The listing builds one solid part. Answer for the finished solid, in the listing's coordinates (mm). A direction names the side the tool comes from. Give positions to 0.01 mm unless a question says otherwise; leave off trailing zeros. Write each loop counter-clockwise with the first axis right and the second up, starting at its lowest first coordinate (ties: lowest second). Pieces come first, ordered by that corner, then holes. Notation, with made-up numbers: (64, 28) - (116, 28) arc R20 ccw to (116, 66) - close; hole circle Ø5 at (0, 53.5). An arc over 180 degrees is marked (long way). Answer in a Markdown table with one row per item. Add a question column.
Autodesk Inventor part; units mm, degrees
ref_plane "YZ Plane" through (0, 0, 0) normal (1, 0, 0) x (0, 1, 0)
ref_plane "XZ Plane" through (0, 0, 0) normal (0, 1, 0) x (-1, 0, 0)
ref_plane "XY Plane" through (0, 0, 0) normal (0, 0, 1) x (1, 0, 0)
sketch "Sketch1" plane through (0, 0, 0) normal (1, 0, 0) x (0, 1, 0)
  line L0 (0, 0) -> (3.95, 0)
  line L1 (3.95, 0) -> (3.95, 0.1833)
  line L2 (3.95, 0.1833) -> (3.7667, 0.3667)
  line L3 (3.7667, 0.3667) -> (3.7667, 0.55)
  line L4 (3.7667, 0.55) -> (6.555, 0.55)
  line L5 (6.555, 0.55) -> (6.555, 1.1)
  line L6 (6.555, 1.1) -> (3.115, 1.1)
  line L7 (3.115, 1.1) -> (3.115, 1.2)
  arc A0 (3.115, 1.3908) -> (3.115, 1.2) centre (3.145, 1.2954) ccw
  line L8 (3.115, 1.6816) -> (3.115, 5.1)
  line L9 (3.115, 5.1) -> (0, 5.1)
  line L10 (0, 5.1) -> (0, 0)
  arc A1 (3.115, 1.6816) -> (3.115, 1.4908) centre (3.145, 1.5862) ccw
  line L11 (3.115, 1.3908) -> (3.115, 1.4908)
  dimension "d0" = 7.9
  dimension "d1" = 1.1
  dimension "d2" = 6.23
  dimension "d3" = 13.11
  dimension "d4" = 4
  dimension "d5" = 0.1
  dimension "d6" = 0.55
  dimension "d7" = 0.1833
  dimension "d8" = 0.1833
  dimension "d9" = 0.1833
  dimension "d10" = 0.03
  dimension "d11" = 0.1
  dimension "d12" = 0.1
revolve "Revolution1" add sketch "Sketch1" angle 360 about axis through (0, 0, 5.1) along (0, 0, -1)
sketch "Sketch2" plane through (0, 0, 0.55) normal (0, 0, -1) x (-1, 0, 0)
  line L0 (1.1709, 4.37) -> (3.1991, 3.1991)
  line L1 (3.1991, 3.1991) -> (4.37, 1.1709)
  line L2 (4.37, 1.1709) -> (4.37, -1.1709)
  line L3 (4.37, -1.1709) -> (3.1991, -3.1991)
  line L4 (3.1991, -3.1991) -> (1.1709, -4.37)
  line L5 (1.1709, -4.37) -> (-1.1709, -4.37)
  line L6 (-1.1709, -4.37) -> (-3.1991, -3.1991)
  line L7 (-3.1991, -3.1991) -> (-4.37, -1.1709)
  line L8 (-4.37, -1.1709) -> (-4.37, 1.1709)
  line L9 (-4.37, 1.1709) -> (-3.1991, 3.1991)
  line L10 (-3.1991, 3.1991) -> (-1.1709, 4.37)
  line L11 (-1.1709, 4.37) -> (1.1709, 4.37)
  circle A0 centre (0, 0) radius 6.555
  dimension "d16" = 8.74
extrude "Extrusion1" cut sketch "Sketch2" against normal through all
hole "Hole1" at (0, 0, 5.1) direction (0, 0, -1) diameter 3.242 end through all countersink diameter 4.2 countersink angle 120
hole "Hole2" [suppressed]
equation "\"d0\" = C_"
equation "\"d1\" = A_"
equation "\"d2\" = B"
equation "\"d3\" = 1.5 * H_"
equation "\"d4\" = Length_Code"
equation "\"d5\" = Mark_1"
equation "\"d6\" = 0.5 * A_"
equation "\"d7\" = 0.166667 * A_"
equation "\"d8\" = 0.166667 * A_"
equation "\"d9\" = 0.166667 * A_"
equation "\"d10\" = Mark_2"
equation "\"d11\" = Mark_1"
equation "\"d12\" = Mark_1"
equation "\"d13\" = T_"
equation "\"d14\" = 1.05 * Thread"
equation "\"d53\" = Length_Code"
equation "\"d18\" = 1.05 * Thread"
equation "\"d20\" = T_"
equation "\"d16\" = H_"
equation "\"Length_Code\" = 4"
equation "\"T_\" = 4"
equation "\"A_\" = 1.1"
equation "\"B\" = 6.23"
equation "\"C_\" = 7.9"
equation "\"H_\" = 8.74"
equation "\"Mark_1\" = 0.1"
equation "\"Mark_2\" = 0.03"
equation "\"Thread\" = 4"
equation "\"Min_Thick\" = 1.6"
equation "\"B_Hole\" = 7.92"
equation "\"Min_Depht\" = 1.1"
equation "\"Min_Dist\" = 6.4"
properties part number "CSS-M4-4" material "Stainless Steel"
1. Section C-C (z = 2.45) is taken. Give the vertices of the cut face in (x, y) (3 decimals), and give its area (3 significant figures).
2. A tool of negligible diameter and unlimited length cuts with its end or side. For faces 4 (the face through (-0.94, 2.97, 3.41)), 5 (the face through (4, -1, 0.55)), 6 (the face through (-2, 0, 0)), from which of +Z, -Z, +X, -X, +Y, -Y can it reach the whole face along a straight path? Write none if from no direction.
3. Straight lines are drawn through the part: L1, parallel to X at y = 0, z = 2.9 (3 decimals); L2, parallel to X at y = 0, z = 0.85; L3, parallel to Z at x = 1.25, y = 3. For each, find the intervals that lie inside material, in ascending order. Write a range as [from, to].
4. Given pin 1 Ø2 at (x, z) = (1, 2.5) entering from +Y (3 decimals); pin 2 Ø1.5 at (y, z) = (-0.5, 3.5) entering from +X (3 decimals); pin 3 Ø1.5 at (x, z) = (-2.5, 3) entering from +Y, each flat-ended and moving along its own axis, determine where each tip first touches the part or whether it passes through.
5. The mould has two halves that part along Y. Classify faces 1 (the face through (1.438, -0.748, 2.378)), 2 (the face through (-2.171, 3.793, 0.821)), 3 (the face through (3.776, -2.199, 0.821)): +Y half, -Y half, draft (parallel to the pull), parting line (faces both ways), or undercut.
Geometry check:
| question | item | result |
|---|---|---|
| 1 | outline | circle Ø6.23 at (0, 0); hole circle Ø3.242 at (0, 0) |
| 1 | area | 22.2 mm² |
| 2 | face 4 | +Z |
| 2 | face 5 | none |
| 2 | face 6 | -Z, +X, -X, +Y, -Y |
| 3 | L1 | [-3.115, -1.621], [1.621, 3.115] |
| 3 | L2 | [-4.37, -1.62], [1.62, 4.37] |
| 3 | L3 | [0, 1.1] |
| 4 | pin 1 | y = 3.115 |
| 4 | pin 2 | x = 3.115 |
| 4 | pin 3 | y = 2.58 |
| 5 | face 1 | undercut |
| 5 | face 2 | +Y half |
| 5 | face 3 | -Y half |
